Read the model definition and answer for the solid it produces. Units are mm, in the model's axes. A direction names the side the tool comes from. Round coordinates to 2 decimals unless told otherwise and drop trailing zeros. Write each loop counter-clockwise with the first axis right and the second up, starting at its lowest first coordinate (ties: lowest second). Pieces come first, ordered by that corner, then holes. Notation, with made-up numbers: M -5,7 L 18,7 A7 cw 18,19 Z; hole C 41,52.5 d11. An arc over 180 degrees is marked long. Use one line per item in the form item = value. Start each with the question number.
Autodesk Inventor part; units mm, degrees
ref_plane "YZ Plane" through (0, 0, 0) normal (1, 0, 0) x (0, 1, 0)
ref_plane "XZ Plane" through (0, 0, 0) normal (0, 1, 0) x (-1, 0, 0)
ref_plane "XY Plane" through (0, 0, 0) normal (0, 0, 1) x (1, 0, 0)
sketch "Sketch1" plane through (0, 0, 0) normal (0, 0, 1) x (1, 0, 0)
  line L0 (0, 0) -> (18, 0)
  line L1 (18, 0) -> (18, 3)
  line L2 (18, 3) -> (0, 3)
  line L3 (0, 3) -> (0, 0)
  line L4 (0, 3) -> (21, 3)
  line L5 (21, 3) -> (21, 2)
  line L6 (21, 2) -> (0, 2)
  line L7 (0, 2) -> (0, 3)
  point P0 (18, 2)
  dimension "d0" = 18
  dimension "d1" = 3
  dimension "d2" = 21
  dimension "d3" = 1
revolve "Revolution1" add sketch "Sketch1" angle 360 about axis through (0, 3, 0) along (0, -1, 0)
mirror "Mirror1" about plane through (0, 0, 0) normal (0, 1, 0) of "Revolution1"
sketch "Sketch2" plane through (0, 3, 0) normal (0, 1, 0) x (1, 0, 0)
  circle A0 centre (0, 0) radius 2.5
  dimension "d5" = 5
extrude "Extrusion1" cut sketch "Sketch2" against normal blind 10
properties part number "servo_pulley"
Q1. Each of these flat-tipped pins is pushed along its axis until it touches: pin 1 Ø1.5 at (x, y) = (12.5, 1.5) entering from +Z; pin 2 Ø1.5 at (x, y) = (15, 0.5) entering from +Z. Where does it stop, or does it pass through?
Q2. Find section B-B on z = 0. Write down the section's boundary in (x, y).
Q3. For a pull along Y with two mould halves and no side action, classify faces 3 (the face through (-0.54, 0.04, 2.44)), 4 (the face through (-9, 2, 16)), 5 (the face through (4, 3, 0)) as +Y half, -Y half, draft (parallel to the pull), parting line (faces both ways), or undercut.
Q4. Find section A-A on x = 0. Write down the section's boundary in (y, z).
Q5. Find section C-C on y = 1.45. Write down the section's boundary in (x, z).
Q6. Straight lines are drawn through the part: line 1 (Y direction, x = -12.5, z = 16.5); line 2 (Z direction, x = 0, y = 1.25); line 3 (X direction, y = 1.3, z = -1.5). For each, find the intervals that lie inside material, in ascending order. Write a range as [from, to].
Q7. A tool of negligible diameter and unlimited length cuts with its end or side. For faces 1 (the face through (20.03, 2.49, 6.31)), 2 (the face through (-2.343, 0.028, -17.847)), from which of +Z, -Z, +X, -X, +Y, -Y can it reach the whole face along a straight path? Write none if from no direction.
Q8. Find section D-D on x = 12.5. Write down the section's boundary in (y, z).
Response:
q1.pin_1 = 17.27
q1.pin_2 = 11
q2.outline = M -21,-3 L -2.5,-3 L -2.5,3 L -21,3 L -21,2 L -18,2 L -18,-2 L -21,-2 Z; M 2.5,-3 L 21,-3 L 21,-2 L 18,-2 L 18,2 L 21,2 L 21,3 L 2.5,3 Z
q3.face_3 = draft
q3.face_4 = undercut
q3.face_5 = +Y half
q4.outline = M -3,-21 L -2,-21 L -2,-18 L 2,-18 L 2,-21 L 3,-21 L 3,-2.5 L -3,-2.5 Z; M -3,2.5 L 3,2.5 L 3,21 L 2,21 L 2,18 L -2,18 L -2,21 L -3,21 Z
q5.outline = C 0,0 d36; hole C 0,0 d5
q6.line_1 = [-3, -2], [2, 3]
q6.line_2 = [-18, -2.5], [2.5, 18]
q6.line_3 = [-17.94, -2], [2, 17.94]
q7.face_1 = +Y, -Y
q7.face_2 = none
q8.outline = M -3,-16.87 L -2,-16.87 L -2,-12.95 L 2,-12.95 L 2,-16.87 L 3,-16.87 L 3,16.87 L 2,16.87 L 2,12.95 L -2,12.95 L -2,16.87 L -3,16.87 Z
